Can you work these out from the model? Positions are in its coordinate system, mm. A direction names the side the tool comes from. Coordinates: 2 decimals unless noted, no trailing zeros. Write each loop counter-clockwise with the first axis right and the second up, starting at its lowest first coordinate (ties: lowest second). Pieces come first, ordered by that corner, then holes. Notation, with made-up numbers: M 38,52.25 L 91,52.25 A25 cw 91,65.25 Z; hole C -21,-29.75 d5. An arc over 180 degrees is marked long. Answer as a JSON object with one key per item and string values. Group by question number.
from build123d import *

# Parameters (mm, degrees)
SKETCH2_R           = 6
BOSS_EXTRUDE1_DEPTH = 12
SKETCH4_R           = 15
BOSS_EXTRUDE3_DEPTH = 30
RIB10_REACH         = 137.185
SKETCH8_WALL_W      = 367.382862114
SKETCH8_WALL_H      = 10


with BuildPart() as part:
    # Sketch2 → Boss-Extrude1 (new body)
    with BuildSketch(Plane(origin=(0, 0, 0), x_dir=(1, 0, 0), z_dir=(0, 1, 0))):
        with BuildLine():
            Line((20, -25), (20, 25))
            ThreePointArc((20, 25), (0, 45), (-20, 25))
            Line((-20, 25), (-20, 15))
            Line((-20, 15), (-70, 15))
            Line((-70, 15), (-70, -15))
            Line((-70, -15), (-20, -15))
            Line((-20, -15), (-20, -25))
            ThreePointArc((-20, -25), (0, -45), (20, -25))
        make_face()
        with Locations(Location((0, 25, 0), (0, 0, 270))):
            Circle(SKETCH2_R, mode=Mode.SUBTRACT)
        with Locations(Location((0, -25, 0), (0, 0, 90))):
            Circle(SKETCH2_R, mode=Mode.SUBTRACT)
    extrude(amount=BOSS_EXTRUDE1_DEPTH)

    # Sketch4 → Boss-Extrude3 (add)
    with BuildSketch(Plane.XY.offset(15)):
        with BuildLine():
            Line((-70, 25), (-70, 12))
            Line((-70, 12), (-45, 12))
            Line((-45, 12), (-45, 60))
            ThreePointArc((-45, 60), (-84.530954843, 80.34333678), (-78.108108108, 36.351351351))
            ThreePointArc((-78.108108108, 36.351351351), (-72.235198346, 31.974858325), (-70, 25))
        make_face()
        with Locations((-70, 60)):
            Circle(SKETCH4_R, mode=Mode.SUBTRACT)
    extrude(amount=-BOSS_EXTRUDE3_DEPTH)

    # Sketch8 wall → Rib10 (add, up to next)
    with BuildSketch(Plane(origin=(-15.260936943, 43.835856736, 0), x_dir=(-0.742235934483, 0.670138655476, 0), z_dir=(-0.670138655476, -0.742235934483, 0)), mode=Mode.PRIVATE) as rib10_sk1:
        Rectangle(SKETCH8_WALL_W, SKETCH8_WALL_H)
    rib10_tool1 = extrude(rib10_sk1.sketch, amount=RIB10_REACH, mode=Mode.PRIVATE) - part.part
    add(rib10_tool1.solids().sort_by_distance((-15.260936943, 43.835856736, 0))[0])


solid = part.part
Q1. If we section it at C-C on y = 73.5: List the corners of the cut face in (x, z) for me.
Q2. We'd pull the mould along Z, two halves only. Please class faces 1 (the flat face through (-66, 43, -15)), 2 (the flat face through (-45, 36, 10)), 3 (the cylindrical face through (0, 6, 31)): pulls with the +Z half, pulls with the -Z half, needs draft (parallel to the pull), parting line crosses it, or undercut.
Q3. If we section it at A-A on z = -22.5: List the corners of the cut face in (x, y) for me, and give its area (3 significant figures).
Q4. Please list where these lines run through material, in increasing order: L1, parallel to X at y = 6, z = 25; L2, parallel to Z at x = -79, y = 73; L3, parallel to Y at x = -62, z = -14.
Q5. If we section it at D-D on z = -8: List the corners of the cut face in (x, y) for me, and give its area (3 significant figures).
Q6. If we section it at B-B on x = 0: List the corners of the cut face in (y, z) for me, and give its area (3 significant figures).
Q7. On a 3-axis mill with a long thin cutter (end or side, diameter ignored), from which of +Z, -Z, +X, -X, +Y, -Y can I reach the whole of each face in a straight line? I mean faces 4 (the flat face through (-45, 36, -10)), 5 (the cylindrical face through (0, 6, -45)), 6 (the flat face through (-70, 13, 0)), 7 (the flat face through (-20, 6, 20)), 8 (the flat face through (-26, 31, 5)). Say none if no direction works.
Q8. Will these pins go through, and if not, where does the flat tip stop? pin 1 (8 mm diameter, centred on y = 37, z = -8, fed in from +X); pin 2 (10 mm diameter, centred on y = 19.5, z = 13.5, fed in from +X); pin 3 (11 mm diameter, centred on y = 3.5, z = -22.5, fed in from -X).
Reply:
{
 "1": {"outline": "M -91.04,-15 L -76.54,-15 L -76.54,15 L -91.04,15 Z; M -63.46,-15 L -48.96,-15 L -48.96,-5 L -48.12,-5 L -48.12,5 L -48.96,5 L -48.96,15 L -63.46,15 Z"},
 "2": {"face 1": "pulls with the -Z half", "face 2": "needs draft", "face 3": "undercut"},
 "3": {"outline": "M -20,0 L -5.45,0 L -5.45,12 L -20,12 Z; M 5.45,0 L 20,0 L 20,12 L 5.45,12 Z", "area": "349 mm^2"},
 "4": {"L1": "-20 to -6, 6 to 20", "L2": "-15 to 15", "L3": "0 to 47.31, 72.69 to 83.69"},
 "5": {"outline": "M -78.11,36.35 A12 cw -70,25 L -70,0 L 20,0 L 20,12 L -45,12 L -45,60 A25 ccw long Z; hole C -70,60 d30", "area": "3,060 mm^2"},
 "6": {"outline": "M 0,-45 L 12,-45 L 12,-31 L 0,-31 Z; M 0,-19 L 12,-19 L 12,-5 L 30.06,-5 L 30.06,5 L 12,5 L 12,19 L 0,19 Z; M 0,31 L 12,31 L 12,45 L 0,45 Z", "area": "973 mm^2"},
 "7": {"face 4": "-Z, +X, +Y", "face 5": "-Z, +Y, -Y", "face 6": "+Z, -Z, -X, -Y", "face 7": "+Z, -X, +Y, -Y", "face 8": "+Z, +X, +Y"},
 "8": {"pin 1": "x = -4.76", "pin 2": "x = -45", "pin 3": "x = -20"}
}
